Here's how the part is built. I have some questions about the finished solid (model axes, mm). A direction names the side the tool comes from. Coordinates: 2 decimals unless noted, no trailing zeros. Loops run counter-clockwise (first coordinate to the right, second up) from the corner with the lowest first, then second, coordinate; pieces in that order, holes last. Notation, with made-up numbers: (27, 8) -> (85, 8) arc R23 cw to (85, 40) -> close; hole circle Ø7 at (80, 53). An arc over 180 degrees is marked (long way). Answer as a JSON object with one key per item and string values. Group by question number.
1) I need wall thicknesses on probe 1 along X at (y, z) = (-15.75, 10); probe 2 along X at (y, z) = (23, 23); probe 3 along X at (y, z) = (-15.5, 30). Which ranges of each line are inside material? Lowest first, please. Write a range as [from, to].
2) I want a section at A-A (z = 20). Write out the boundary of the cut face in (x, y).
3) Which directions (+Z, -Z, +X, -X, +Y, -Y) give clear straight access to the entire face, cutting with the end or side of a thin tool? Please do faces 4 (the flat face through (-14, -10, 2)), 5 (the cylindrical face through (-26.419, 18.887, 8.452)), 6 (the flat face through (20, 20, 22)).
4) I want a section at D-D (z = 4). Write out the boundary of the cut face in (x, y), then the cut area to 3 significant figures.
5) I'm going to push flat-ended pins straight in: pin 1 (5 mm diameter, centred on x = -12.02, y = 12.02, fed in from +Z); pin 2 (2.5 mm diameter, centred on x = -25, z = 10, fed in from +Y); pin 3 (9 mm diameter, centred on x = -12, y = -11.5, fed in from +Z); pin 4 (3.5 mm diameter, centred on x = 12.02, y = -12.02, fed in from -Z). Where does each tip first touch, or does it pass through?
6) I want a section at B-B (x = 0). Write out the boundary of the cut face in (y, z), then the cut area to 3 significant figures.
7) If we mould it in two halves opening along Z, with no side actions, what happens to faces 1 (the conical face through (25.222, 11.557, 9.711)), 2 (the flat face through (-26, 0, 38)), 3 (the cylindrical face through (10.08, 11.22, 0.99))? For each: +Z half, -Z half, draft (parallel to the pull), parting line (faces both ways), or undercut.
8) I want a section at C-C (y = 0). Write out the boundary of the cut face in (x, z).
```python
from build123d import *

# Parameters (mm, degrees)
SKETCH_1_W                  = 60
SKETCH_1_H                  = 50
EXTRUDE_1_DEPTH             = 38
SKETCH_2_W                  = 40
SKETCH_2_H                  = 67.456297037
CUT_EXTRUDE_1_DEPTH         = 70.598850565
SKETCH_3_R                  = 25
CUT_EXTRUDE_2_DEPTH         = 32
SKETCH_4_R                  = 13.25
CUT_EXTRUDE_3_DEPTH         = 10
HOLE_WIZARD_4_2_4_2_1_D     = 4.2
HOLE_WIZARD_M5_2_AT_2_COUNT = 2
HOLE_WIZARD_M5_2_AT_2_PITCH = 50
SKETCH_11_R                 = 4
CUT_EXTRUDE_4_DEPTH         = 4
PATTERN_CIRCULAR_1_COUNT    = 4


with BuildPart() as part:
    # 草图1 → 凸台-拉伸1 (new body)
    with BuildSketch(Plane.XY):
        Rectangle(SKETCH_1_W, SKETCH_1_H)
    extrude(amount=EXTRUDE_1_DEPTH)

    # 草图2 → 切除-拉伸1 (cut, through all)
    with BuildSketch(Plane(origin=(0, 25, 0), x_dir=(1, 0, 0), z_dir=(0, 1, 0))):
        with Locations((0, -39.728148518)):
            Rectangle(SKETCH_2_W, SKETCH_2_H)
    extrude(amount=-CUT_EXTRUDE_1_DEPTH, mode=Mode.SUBTRACT)

    # 草图3 → 切除-拉伸2 (cut)
    with BuildSketch(Plane.XY.offset(38)):
        Circle(SKETCH_3_R)
    extrude(amount=-CUT_EXTRUDE_2_DEPTH, mode=Mode.SUBTRACT)

    # 草图4 → 切除-拉伸3 (cut)
    with BuildSketch(Plane(origin=(0, 0, 0), x_dir=(-1, 0, 0), z_dir=(0, 0, -1))):
        Circle(SKETCH_4_R)
    extrude(amount=-CUT_EXTRUDE_3_DEPTH, mode=Mode.SUBTRACT)

    # Ø4.2 (4.2) 直径孔1 (through all)
    with Locations(Plane.XY.offset(6)):
        with Locations((12.02081528, 12.02081528), (-12.02081528, 12.02081528), (-12.02081528, -12.02081528), (12.02081528, -12.02081528)):
            Hole(HOLE_WIZARD_4_2_4_2_1_D / 2)

    # 草图7 → M5 螺纹孔1 (revolve, cut)
    with BuildSketch(Plane(origin=(25, 14, 38), x_dir=(0, -1, 0), z_dir=(1, 0, 0))):
        Polygon((0, 0), (0, 23.6618073), (2.1, 22.4), (2.1, 0), align=None)
    hole_wizard_m5_1 = revolve(axis=Axis((25, 14, 44.35), (0, 0, -1)), mode=Mode.SUBTRACT)

    # 镜向1: M5 螺纹孔1 across plane
    add(hole_wizard_m5_1.mirror(Plane.ZX), mode=Mode.SUBTRACT)

    # 镜向2: M5 螺纹孔1 across plane
    add(hole_wizard_m5_1.mirror(Plane.ZY), mode=Mode.SUBTRACT)

    # 镜向2 copy 1 sketch → 镜向2 copy 1 (revolve, cut)
    with BuildSketch(Plane(origin=(-25, -14, 38), x_dir=(0, 1, 0), z_dir=(-1, 0, 0))):
        Polygon((0, 0), (0, 23.6618073), (2.1, 22.4), (2.1, 0), align=None)
    revolve(axis=Axis((-25, -14, 44.35), (0, 0, -1)), mode=Mode.SUBTRACT)

    # 草图9 → M5 螺纹孔2 (revolve, cut)
    with BuildSketch(Plane(origin=(-25, 25, 10), x_dir=(0, 0, 1), z_dir=(1, 0, 0))):
        Polygon((0, 0), (0, 13.6618073), (2.1, 12.4), (2.1, 0), align=None)
    hole_wizard_m5_2 = revolve(axis=Axis((-25, 31.35, 10), (0, -1, 0)), mode=Mode.SUBTRACT)

    # M5 螺纹孔2 at 2: M5 螺纹孔2 ×2
    with Locations(*[(i * HOLE_WIZARD_M5_2_AT_2_PITCH, 0, 0) for i in range(1, HOLE_WIZARD_M5_2_AT_2_COUNT)]):
        add(hole_wizard_m5_2, mode=Mode.SUBTRACT)

    # 镜向3: M5 螺纹孔2 across plane
    add(hole_wizard_m5_2.mirror(Plane.ZX), mode=Mode.SUBTRACT)

    # 镜向3 copy 1 sketch → 镜向3 copy 1 (revolve, cut)
    with BuildSketch(Plane(origin=(25, -25, 10), x_dir=(0, 0, 1), z_dir=(1, 0, 0))):
        Polygon((0, 0), (0, -13.6618073), (2.1, -12.4), (2.1, 0), align=None)
    revolve(axis=Axis((25, -31.35, 10), (0, -1, 0)), mode=Mode.SUBTRACT)

    # 草图11 → 切除-拉伸4 (cut)
    with BuildSketch(Plane.XY.offset(6)):
        with Locations((12.02081528, 12.02081528)):
            Circle(SKETCH_11_R)
    cut_extrude_4 = extrude(amount=-CUT_EXTRUDE_4_DEPTH, mode=Mode.SUBTRACT)

    # 阵列(圆周)1: 切除-拉伸4 ×4 about axis
    pattern_circular_1_axis = Axis((0, 0, 0), (0, 0, 1))
    for i in range(1, PATTERN_CIRCULAR_1_COUNT):
        add(cut_extrude_4.rotate(pattern_circular_1_axis, i * 360 / PATTERN_CIRCULAR_1_COUNT), mode=Mode.SUBTRACT)


solid = part.part
```
Determined:
{
 "1": {"probe 1": "[-30, -27.1], [-22.9, -20], [20, 22.9], [27.1, 30]", "probe 2": "[-30, -20], [20, 30]", "probe 3": "[-30, -26.47], [-23.53, -20], [20, 23.53], [26.47, 30]"},
 "2": {"outline": "(-30, -25) -> (-20, -25) -> (-20, -15) arc R25 cw to (-20, 15) -> (-20, 25) -> (-30, 25) -> close; (20, -25) -> (30, -25) -> (30, 25) -> (20, 25) -> (20, 15) arc R25 cw to (20, -15) -> close; hole circle Ø4.2 at (-25, -14); hole circle Ø4.2 at (-25, 14); hole circle Ø4.2 at (25, -14); hole circle Ø4.2 at (25, 14)"},
 "3": {"face 4": "+Z", "face 5": "+Y", "face 6": "+Z, +Y, -Y"},
 "4": {"outline": "(-30, -25) -> (30, -25) -> (30, 25) -> (-30, 25) -> close; hole (-10.2, -8.46) arc R4 ccw (long way) to (-8.46, -10.2) arc R13.25 ccw to (8.46, -10.2) arc R4 ccw (long way) to (10.2, -8.46) arc R13.25 ccw to (10.2, 8.46) arc R4 ccw (long way) to (8.46, 10.2) arc R13.25 ccw to (-8.46, 10.2) arc R4 ccw (long way) to (-10.2, 8.46) arc R13.25 ccw to start", "area": "2,250 mm^2"},
 "5": {"pin 1": "z = 2", "pin 2": "y = 12.09", "pin 3": "z = 6", "pin 4": "through"},
 "6": {"outline": "(-25, 0) -> (-13.25, 0) -> (-13.25, 6) -> (-25, 6) -> close; (13.25, 0) -> (25, 0) -> (25, 6) -> (13.25, 6) -> close", "area": "141 mm^2"},
 "7": {"face 1": "undercut", "face 2": "+Z half", "face 3": "draft"},
 "8": {"outline": "(-30, 0) -> (-13.25, 0) -> (-13.25, 6) -> (-25, 6) -> (-25, 38) -> (-30, 38) -> close; (13.25, 0) -> (30, 0) -> (30, 38) -> (25, 38) -> (25, 6) -> (13.25, 6) -> close"}
}
